Model file for the job. Use its own axes, mm. Round coordinates to 2 decimals unless told otherwise and drop trailing zeros. Loops run counter-clockwise (first coordinate to the right, second up) from the corner with the lowest first, then second, coordinate; pieces in that order, holes last. Notation, with made-up numbers: M 89.25,-6.5 L 144.25,-6.5 A25 cw 144.25,15.5 Z; hole C 28.25,41 d1. An arc over 180 degrees is marked long. Answer in a Markdown table with one row per item.
from build123d import *

# Parameters (mm, degrees)
SKETCH_W     = 25
SKETCH_H     = 23
PAD_DEPTH    = 1.5
SKETCH001_W  = 15.7
SKETCH001_H  = 17
POCKET_DEPTH = 5
SKETCH002_W  = 1.5
SKETCH002_H  = 1.5
PAD001_DEPTH = 2


with BuildPart() as part:
    # Sketch → Pad (new body)
    with BuildSketch(Plane.XY):
        Rectangle(SKETCH_W, SKETCH_H)
    extrude(amount=PAD_DEPTH)

    # Sketch001 (on Face6 of Pad) → Pocket (cut)
    with BuildSketch(Plane.XY.offset(1.5)):
        with Locations((0, -3)):
            Rectangle(SKETCH001_W, SKETCH001_H)
    extrude(amount=-POCKET_DEPTH, mode=Mode.SUBTRACT)

    # Sketch002 (on Face4 of Pocket) → Pad001 (join)
    with BuildSketch(Plane(origin=(0, 0, 1.5), x_dir=(1, 0, 0), z_dir=(0, 0, -1))):
        with Locations((-8.6, 2.5)):
            Rectangle(SKETCH002_W, SKETCH002_H)
    extrude(amount=-PAD001_DEPTH)


solid = part.part
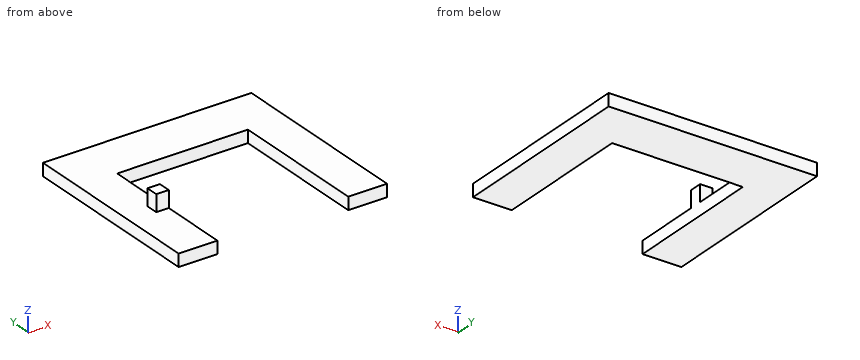
1. Wall check: probe 1 along Y at (x, z) = (7, 0.8); probe 2 along Z at (x, y) = (9, 9); probe 3 along X at (y, z) = (-9.5, 0.2). Give the ranges that are in metal, low to high.
Verdict:
| item | result |
|---|---|
| probe 1 | y = 5.5 to 11.5 |
| probe 2 | z = 0 to 1.5 |
| probe 3 | x = -12.5 to -7.85, 7.85 to 12.5 |
2. Saw through at C-C (x = -10). Write the cut outline in (y, z).
Verdict:
| item | result |
|---|---|
| outline | M -11.5,0 L 11.5,0 L 11.5,1.5 L -11.5,1.5 Z |
3. Saw through at B-B (z = 0.95). Write the cut outline in (x, y), and give its area (3 significant figures).
Verdict:
| item | result |
|---|---|
| outline | M -12.5,-11.5 L -7.85,-11.5 L -7.85,5.5 L 7.85,5.5 L 7.85,-11.5 L 12.5,-11.5 L 12.5,11.5 L -12.5,11.5 Z |
| area | 308 mm² |
4. Saw through at D-D (y = 7.25). Write the cut outline in (x, z).
Verdict:
| item | result |
|---|---|
| outline | M -12.5,0 L 12.5,0 L 12.5,1.5 L -12.5,1.5 Z |
5. Saw through at A-A (y = 1.75). Write the cut outline in (x, z).
Verdict:
| item | result |
|---|---|
| outline | M -12.5,0 L -7.85,0 L -7.85,1.5 L -12.5,1.5 Z; M 7.85,0 L 12.5,0 L 12.5,1.5 L 7.85,1.5 Z |
6. Pin check, flat tips, straight feed: pin 1 (10 mm diameter, centred on x = 9.5, y = 8, fed in from +Z); pin 2 (1.5 mm diameter, centred on x = -5, z = 0.5, fed in from -Y); pin 3 (12 mm diameter, centred on x = -7, y = 1.5, fed in from +Z); pin 4 (0.8 mm diameter, centred on x = -9, z = 2.5, fed in from -Y). Stop position of each tip, or through.
Verdict:
| item | result |
|---|---|
| pin 1 | stops at z = 1.5 |
| pin 2 | stops at y = 5.5 |
| pin 3 | stops at z = 3.5 |
| pin 4 | stops at y = -3.25 |
